Design review of the part built by this model. Coordinates are the model's own, in mm. A direction names the side the tool comes from. Coordinates: 2 decimals unless noted, no trailing zeros. Loops run counter-clockwise (first coordinate to the right, second up) from the corner with the lowest first, then second, coordinate; pieces in that order, holes last. Notation, with made-up numbers: (25, 5.25) - (32, 5.25) arc R26 ccw to (32, 34.25) - close; hole circle Ø4 at (86.5, -37). An arc over 180 degrees is marked (long way). Answer in a Markdown table with one row per item. Add a question column.
(1) To check wall thickness, follow L1, parallel to Y at x = 0.7, z = 2.5; L2, parallel to Y at x = 3.3, z = 2.5; L3, parallel to Y at x = 3.65, z = 4.2. State the ranges of each line that lie inside material, in increasing order. Write a range as [from, to].
(2) We need section D-D, the plane x = 1.05. Write out the cut boundary in (y, z), plus the area to 3 significant figures.
(3) We need section C-C, the plane z = 2.5. Write out the cut boundary in (x, y), plus the area to 3 significant figures.
(4) We need section A-A, the plane y = -10. Write out the cut boundary in (x, z), plus the area to 3 significant figures.
(5) For faces 4 (the face through (3, -7, 2)), 5 (the face through (0, -12.4, 2.5)), list the 3-axis set-ups (+Z, -Z, +X, -X, +Y, -Y) from which the entire face can be reached by the end or side of a thin tool; tool diameter is ignored.
(6) Clearance check with flat-ended pins moving along their axes: pin 1 (3 mm diameter, centred on y = -10, z = 2.5, fed in from -X); pin 2 (2.5 mm diameter, centred on y = -4.5, z = 2.5, fed in from +X); pin 3 (1.2 mm diameter, centred on y = -10, z = 2.5, fed in from -X). State where each tip first meets the part, or that it passes through.
(7) The part is to be moulded in two halves that separate along Z. For faces 1 (the face through (0.986, -8.017, 2.24)), 2 (the face through (2, -10, 0)), 3 (the face through (2, 0, 2)), say which applies: released by +Z, released by -Z, zero draft, split by the parting line, or undercut.
(8) We need section B-B, the plane x = 3.4. Write out the cut boundary in (y, z), plus the area to 3 significant figures.
Autodesk Inventor part; units mm, degrees
ref_plane "YZ Plane" through (0, 0, 0) normal (1, 0, 0) x (0, 1, 0)
ref_plane "XZ Plane" through (0, 0, 0) normal (0, 1, 0) x (-1, 0, 0)
ref_plane "XY Plane" through (0, 0, 0) normal (0, 0, 1) x (1, 0, 0)
sketch "Sketch1" plane through (0, 0, 0) normal (0, 0, 1) x (1, 0, 0)
  line L0 (0, 0) -> (4, 0)
  line L1 (4, 0) -> (4, -20)
  line L2 (4, -20) -> (0, -20)
  line L3 (0, -20) -> (0, 0)
  circle A0 centre (4, -4) radius 2.5
  circle A1 centre (4, -16) radius 2.5
  line L4 (1.5, -4) -> (1.5, -7)
  line L5 (1.5, -7) -> (1.5, -1)
  line L6 (4, -7) -> (1.5, -7)
  line L7 (1.5, -1) -> (4, -1)
  point P0 (4, -18.5)
  point P1 (4, -13.5)
  dimension "d2" = 5
  dimension "d0" = 20
  dimension "d1" = 4
  dimension "d3" = 5
  dimension "d4" = 4
  dimension "d5" = 4
  dimension "d6" = 3
  dimension "d7" = 3
extrude "Extrusion1" add sketch "Sketch1" along normal blind 5 contours L0 L1 L7 L5 L4 L6 A1 L2 L3
sketch "Sketch3" plane through (0, -20, 0) normal (-1, 0, 0) x (0, 0, 1)
  circle A0 centre (2.5, 10) radius 1.35
  line L0 (0, 0) -> (5, 0)
  line L1 (0, 20) -> (0, 0)
  dimension "d10" = 10
  dimension "d11" = 2.5
  dimension "d12" = 20
  dimension "d13" = 2.7
extrude "Extrusion2" cut sketch "Sketch3" against normal blind 20
sketch "Sketch4" plane through (0, -20, 0) normal (-1, 0, 0) x (0, 0, 1)
  circle A0 centre (2.5, 10) radius 1.35
  circle A1 centre (2.5, 10) radius 2
  point P0 (0, 20)
  dimension "d16" = 4
extrude "Extrusion3" cut sketch "Sketch4" against normal blind 2 contours A0 | A1
equation "\"d1\" = d4"
properties part number "POMSliderAxis"
Responses:
| question | item | result |
|---|---|---|
| 1 | L1 | y = [-20, -12], [-8, 0] |
| 1 | L2 | y = [-20, -18.4], [-13.6, -11.35], [-8.65, -7], [-1, 0] |
| 1 | L3 | y = [-20, -18.48], [-13.52, -7], [-1, 0] |
| 2 | outline | (-20, 0) - (0, 0) - (0, 5) - (-20, 5) - close; hole circle Ø4 at (-10, 2.5) |
| 2 | area | 87.4 mm2 |
| 3 | outline | (0, -20) - (4, -20) - (4, -18.5) arc R2.5 cw to (4, -13.5) - (4, -11.35) - (2, -11.35) - (2, -12) - (0, -12) - close; (0, -8) - (2, -8) - (2, -8.65) - (4, -8.65) - (4, -7) - (1.5, -7) - (1.5, -1) - (4, -1) - (4, 0) - (0, 0) - close |
| 3 | area | 41.8 mm2 |
| 4 | outline | (0, 0) - (4, 0) - (4, 1.15) - (2, 1.15) - (2, 0.5) - (0, 0.5) - close; (0, 4.5) - (2, 4.5) - (2, 3.85) - (4, 3.85) - (4, 5) - (0, 5) - close |
| 4 | area | 6.60 mm2 |
| 5 | face 4 | +Z, -Z, +X |
| 5 | face 5 | +Z, -Z, -X, +Y, -Y |
| 6 | pin 1 | stops at x = 2 |
| 6 | pin 2 | stops at x = 1.5 |
| 6 | pin 3 | passes through |
| 7 | face 1 | undercut |
| 7 | face 2 | released by -Z |
| 7 | face 3 | zero draft |
| 8 | outline | (-20, 0) - (-18.43, 0) - (-18.43, 5) - (-20, 5) - close; (-13.57, 0) - (-7, 0) - (-7, 5) - (-13.57, 5) - close; (-1, 0) - (0, 0) - (0, 5) - (-1, 5) - close; hole circle Ø2.7 at (-10, 2.5) |
| 8 | area | 40.0 mm2 |
